from build123d import *

# Parameters (mm, degrees)
F0_W     = 400
F0_H     = 400
F1_DEPTH = 4
F2_W     = 40
F2_H     = 40
F3_DEPTH = 770
F4_W     = 200
F4_H     = 40
F5_DEPTH = 4
F8_D     = 20
F8_DEPTH = 20
F9_D     = 20
F9_DEPTH = 20


with BuildPart() as f1:
    # F0 (on Top) → F1 (new body)
    with BuildSketch(Plane.XY):
        Rectangle(F0_W, F0_H)
    extrude(amount=F1_DEPTH)

    # F2 (on face) → F3 (join)
    with BuildSketch(Plane.XY.offset(4)):
        Rectangle(F2_W, F2_H)
    extrude(amount=F3_DEPTH)

    # F4 (on face) → F5 (join)
    with BuildSketch(Plane.XY.offset(774)):
        Rectangle(F4_W, F4_H)
    extrude(amount=F5_DEPTH)

    # F8
    with Locations(Plane.XY.offset(778)):
        with Locations((-65, 0)):
            Hole(F8_D / 2, depth=F8_DEPTH)

    # F9
    with Locations(Plane.XY.offset(778)):
        with Locations((65, 0)):
            Hole(F9_D / 2, depth=F9_DEPTH)


solid = f1.part
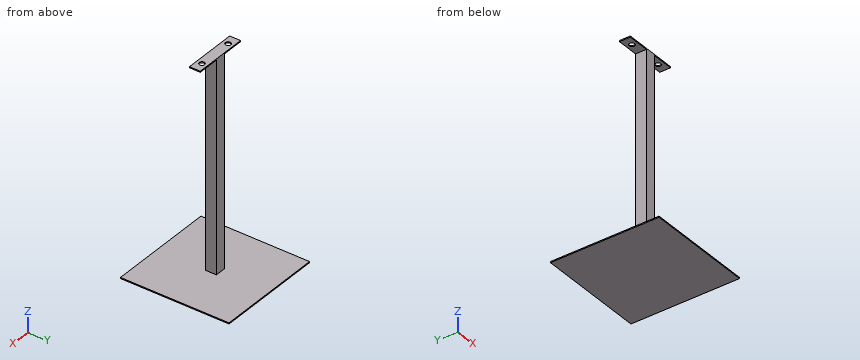
Work out the finished part from the listing and answer in its coordinate system (mm). Give positions to 0.01 mm unless a question says otherwise; leave off trailing zeros. Loops run counter-clockwise (first coordinate to the right, second up) from the corner with the lowest first, then second, coordinate; pieces in that order, holes last. Notation, with made-up numbers: M -35.5,-20.75 L -23.5,-20.75 A24 ccw -23.5,-7.75 Z; hole C 9.25,50.5 d5. An arc over 180 degrees is marked long. Use CSV: the item, a comma, the result in double quotes.
1) Consider L1, parallel to Y at x = -65, z = 776; L2, parallel to Z at x = 122.5, y = -8; L3, parallel to Z at x = -65.5, y = 15.5. Determine where each line is inside the solid, lowest interval first.
Answer:
L1,"-20 to -10, 10 to 20"
L2,"0 to 4"
L3,"0 to 4, 774 to 778"
2) Find section D-D on z = 138. Write down the section's boundary in (x, y), plus the area to 3 significant figures.
Answer:
outline,"M -20,-20 L 20,-20 L 20,20 L -20,20 Z"
area,"1,600 mm^2"
3) Find section A-A on y = 0. Write down the section's boundary in (x, z).
Answer:
outline,"M -200,0 L 200,0 L 200,4 L 20,4 L 20,774 L 55,774 L 55,778 L -55,778 L -55,774 L -20,774 L -20,4 L -200,4 Z; M -100,774 L -75,774 L -75,778 L -100,778 Z; M 75,774 L 100,774 L 100,778 L 75,778 Z"
4) Find section B-B on x = 65. Write down the section's boundary in (y, z), plus the area to 3 significant figures.
Answer:
outline,"M -200,0 L 200,0 L 200,4 L -200,4 Z; M -20,774 L -10,774 L -10,778 L -20,778 Z; M 10,774 L 20,774 L 20,778 L 10,778 Z"
area,"1,680 mm^2"
5) Find section C-C on y = -142.5. Write down the section's boundary in (x, z).
Answer:
outline,"M -200,0 L 200,0 L 200,4 L -200,4 Z"
6) Given P1, Ø4.5, axis at y = 9.5, z = 776, coming from the +X side; P2, Ø20, axis at y = 5, z = 203, coming from the +X side; P3, Ø2, axis at y = -1.5, z = 776.5, coming from the -X side, each flat-ended and moving along its own axis, determine where each tip first touches the part or whether it passes through.
Answer:
P1,"x = 100"
P2,"x = 20"
P3,"x = -100"
